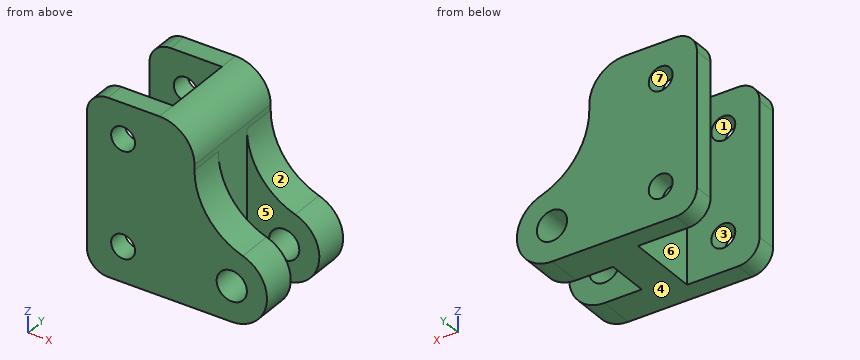
```python
from build123d import *

# Parameters (mm, degrees)
EXTRUDE_1_DEPTH     = 25
SKETCH_2_R          = 1.7
CUT_EXTRUDE_1_DEPTH = 32.369132918
SKETCH_3_R          = 2.15
EXTRUDE_2_DEPTH     = 16
SKETCH_4_W          = 20
SKETCH_4_H          = 6
CUT_EXTRUDE_2_DEPTH = 31.382396219
FILLET_1_R          = 10
FILLET_2_R          = 5
FILLET_3_R          = 3


# Some blends are built 0.0001 mm under size
with BuildPart() as part:
    # ｽｹｯﾁ1 → ﾎﾞｽ - 押し出し1 (new body)
    with BuildSketch(Plane.XY):
        Polygon((5.15, 0), (10.15, 0), (10.15, 8), (-5.15, 8), (-5.15, 5.15), (5.15, 5.15), align=None)
        Polygon((10.15, -8), (10.15, 0), (5.15, 0), (5.15, -5.15), (-5.15, -5.15), (-5.15, -8), align=None)
    extrude(amount=EXTRUDE_1_DEPTH)

    # ｽｹｯﾁ2 → ｶｯﾄ - 押し出し1 (cut, through all)
    with BuildSketch(Plane.XZ.offset(8)):
        with Locations(Location((0, 20, 0), (0, 0, 270))):
            Circle(SKETCH_2_R)
        with Locations(Location((0, 5, 0), (0, 0, 270))):
            Circle(SKETCH_2_R)
    extrude(amount=-CUT_EXTRUDE_1_DEPTH, mode=Mode.SUBTRACT)

    # ｽｹｯﾁ3 → ﾎﾞｽ - 押し出し2 (add, through all)
    with BuildSketch(Plane.XZ.offset(8)):
        with BuildLine():
            Line((10.15, 0), (15.45, 0))
            ThreePointArc((15.45, 0), (20.45, 5), (15.45, 10))
            Line((15.45, 10), (10.15, 10))
            Line((10.15, 10), (10.15, 0))
        make_face()
        with Locations(Location((15.45, 5, 0), (0, 0, 270))):
            Circle(SKETCH_3_R, mode=Mode.SUBTRACT)
    extrude(amount=-EXTRUDE_2_DEPTH)

    # ｽｹｯﾁ4 → ｶｯﾄ - 押し出し2 (cut, through all)
    with BuildSketch(Plane(origin=(10.15, 0, 0), x_dir=(0, 0, -1), z_dir=(1, 0, 0))):
        Rectangle(SKETCH_4_W, SKETCH_4_H)
    extrude(amount=CUT_EXTRUDE_2_DEPTH, mode=Mode.SUBTRACT)

    # ﾌｨﾚｯﾄ1
    # the kernel refuses this fillet: 10 mm, written as the material it adds along each edge
    with BuildSketch(Plane(origin=(10.15, -8, 10), x_dir=(0, 0, 1), z_dir=(0, 1, 0)), Plane(origin=(10.15, 3, 10), x_dir=(0, 0, 1), z_dir=(0, 1, 0))) as fillet_1_piece_1:
        with BuildLine():
            CenterArc((9.244648118, 10), FILLET_1_R, 198.260227933, 71.739772067)
            Line((-0.251783961, 6.866666667), (-1.201427169, 6.553333333))
            ThreePointArc((-1.201427169, 6.553333333), (-1, 5.3), (-1, 0))
            Line((-1, 0), (0, -1))
            Line((0, -1), (9.244648118, -1))
            Line((9.244648118, -1), (9.244648118, 0))
        make_face()
    extrude(amount=5)
    with BuildSketch(Plane(origin=(10.15, -8, 10), x_dir=(0, 0, 1), z_dir=(0, 1, 0))) as fillet_1_piece_2_section:
        with BuildLine():
            CenterArc((9.244648118, 10), FILLET_1_R, 198.260227933, 71.739772067)
            Line((-0.251783961, 6.866666667), (-1.201427169, 6.553333333))
            ThreePointArc((-1.201427169, 6.553333333), (-1, 5.3), (-1, 0))
            Line((-1, 0), (0, -1))
            Line((0, -1), (9.244648118, -1))
            Line((9.244648118, -1), (9.244648118, 0))
        make_face()
    fillet_1_piece_2 = extrude(amount=28.111620295, mode=Mode.PRIVATE)
    fillet_1_piece_2 = split(fillet_1_piece_2, bisect_by=Plane(origin=(11.517519747, 8, 12.315903655), z_dir=(0, -1, 0)), keep=Keep.TOP, mode=Mode.PRIVATE)
    fillet_1_piece_2 = split(fillet_1_piece_2, bisect_by=Plane(origin=(11.517519747, 3, 12.315903655), z_dir=(0, 1, 0)), keep=Keep.TOP, mode=Mode.PRIVATE)
    add(fillet_1_piece_2)
    with BuildSketch(Plane(origin=(10.15, -20.111620295, 10), x_dir=(0, 0, 1), z_dir=(0, 1, 0))) as fillet_1_piece_3_section:
        with BuildLine():
            CenterArc((9.244648118, 10), FILLET_1_R, 198.260227933, 71.739772067)
            Line((-0.251783961, 6.866666667), (-1.201427169, 6.553333333))
            ThreePointArc((-1.201427169, 6.553333333), (-1, 5.3), (-1, 0))
            Line((-1, 0), (0, -1))
            Line((0, -1), (9.244648118, -1))
            Line((9.244648118, -1), (9.244648118, 0))
        make_face()
    fillet_1_piece_3 = extrude(amount=28.111620295, mode=Mode.PRIVATE)
    fillet_1_piece_3 = split(fillet_1_piece_3, bisect_by=Plane(origin=(11.517519747, -8, 12.315903655), z_dir=(0, 1, 0)), keep=Keep.TOP, mode=Mode.PRIVATE)
    fillet_1_piece_3 = split(fillet_1_piece_3, bisect_by=Plane(origin=(11.517519747, -3, 12.315903655), z_dir=(0, -1, 0)), keep=Keep.TOP, mode=Mode.PRIVATE)
    add(fillet_1_piece_3)

    # ﾌｨﾚｯﾄ2
    fillet_2_edges = [part.edges().sort_by_distance(p)[0] for p in [
        (10.15, 0, 25),
    ]]
    fillet(fillet_2_edges, radius=FILLET_2_R - 0.0001)  # a hair under: the kernel refuses the full size

    # ﾌｨﾚｯﾄ3
    fillet_3_edges = [part.edges().sort_by_distance(p)[0] for p in [
        (-5.15, 6.575, 0),
        (-5.15, -6.575, 0),
        (-5.15, -6.575, 25),
        (-5.15, 6.575, 25),
    ]]
    fillet(fillet_3_edges, radius=FILLET_3_R)


solid = part.part
```
Source: CAD feature listing. Evaluate the final solid. Frame: model axes, mm. Face numbers are marked on the shaded views. A direction names the side the tool comes from. Give positions to 0.01 mm unless a question says otherwise; leave off trailing zeros. Order: outer loops, then holes, each group sorted by start corner. A loop starts at its lowest first (then second) coordinate and runs counter-clockwise, first axis right, second up.
(1) Material intervals for line 1 along X through (y, z) = (6.6, 5); line 2 along Y through (x, z) = (15, 10.5); line 3 along Y through (x, z) = (-3, 17.5), sorted ascending.
(2) Pull-direction query (X, two-part tool) for the marked faces 1, 2, 3 and 4; classes: +X half, -X half, draft (parallel to the pull), parting line (faces both ways), or undercut.
(3) Section query A-A (z = 5). Return the cut outline in (x, y).
(4) Access query for the marked faces 5, 6 and 7. Directions: +Z, -Z, +X, -X, +Y, -Y. A direction counts if a zero-diameter tool reaches every point of the face in a straight line with its end or side. Return the directions, or none.
(5) Contact query for a flat-ended pin moving along its axis: P1, Ø5, axis at y = 0, z = 9.5, coming from the -X side. Output: stop coordinate, or through.
(6) Section query B-B (x = 0). Return the cut outline in (y, z).
Outcome:
1. line 1: x = -5.15 to -1.7, 1.7 to 13.3, 17.6 to 20.45
1. line 2: y = -8 to -3, 3 to 8
1. line 3: y = -8 to -5.15, 5.15 to 8
2. face 1: undercut
2. face 2: +X half
2. face 3: undercut
2. face 4: draft
3. outline: (-5.15, -8) - (-1.7, -8) - (-1.7, -5.15) - (-5.15, -5.15) - close; (-5.15, 5.15) - (-1.7, 5.15) - (-1.7, 8) - (-5.15, 8) - close; (1.7, -8) - (13.3, -8) - (13.3, -3) - (10.15, -3) - (10.15, 3) - (13.3, 3) - (13.3, 8) - (1.7, 8) - (1.7, 5.15) - (5.15, 5.15) - (5.15, -5.15) - (1.7, -5.15) - close; (17.6, -8) - (20.45, -8) - (20.45, -3) - (17.6, -3) - close; (17.6, 3) - (20.45, 3) - (20.45, 8) - (17.6, 8) - close
4. face 5: +Z, -Z, +X
4. face 6: +Z, -Z, -X
4. face 7: +Y, -Y
5. P1: stops at x = 5.15
6. outline: (-8, 0) - (-5.15, 0) - (-5.15, 3.3) - (-8, 3.3) - close; (-8, 6.7) - (-5.15, 6.7) - (-5.15, 18.3) - (-8, 18.3) - close; (-8, 21.7) - (-5.15, 21.7) - (-5.15, 25) - (-8, 25) - close; (5.15, 0) - (8, 0) - (8, 3.3) - (5.15, 3.3) - close; (5.15, 6.7) - (8, 6.7) - (8, 18.3) - (5.15, 18.3) - close; (5.15, 21.7) - (8, 21.7) - (8, 25) - (5.15, 25) - close
